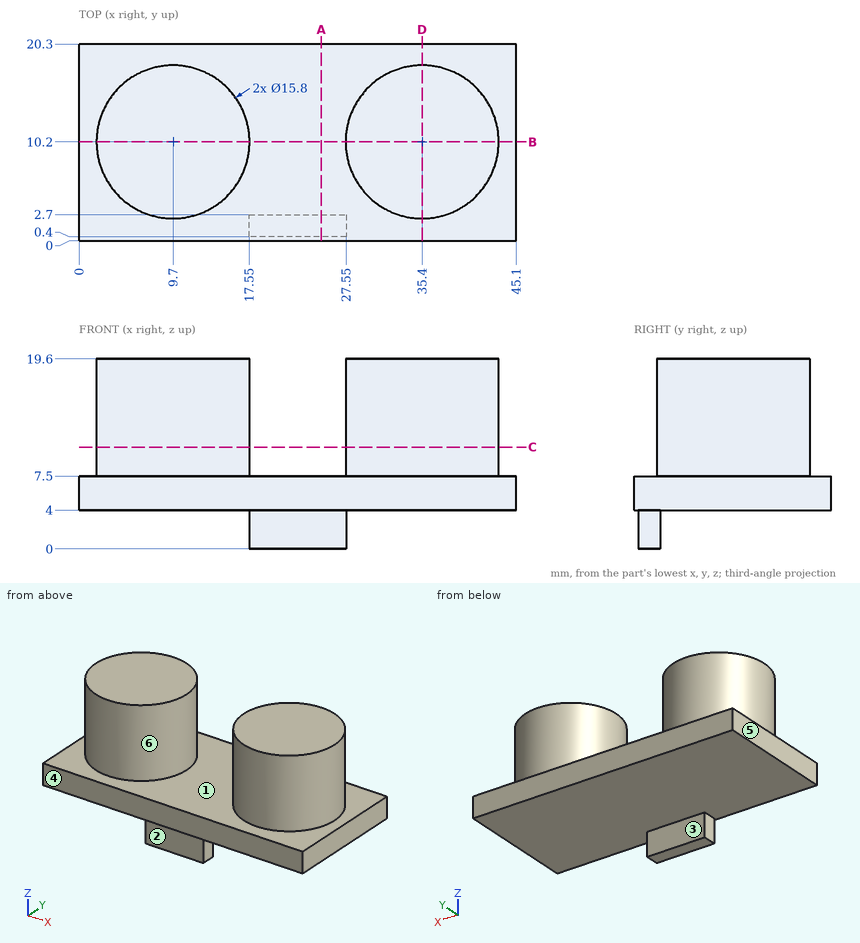
Geometry: see drawing. Coordinates: mm, zero at the bounding-box minimum. A direction names the side the tool comes from. Give positions to 0.01 mm unless a question says otherwise; leave off trailing zeros. Write each loop counter-clockwise with the first axis right and the second up, starting at its lowest first coordinate (ties: lowest second). Pieces come first, ordered by that corner, then holes. Notation, with made-up numbers: (0, 73.25) - (40, 73.25) arc R12 ccw to (40, 89.25) - close; hole circle Ø4 at (38, 16). An arc over 180 degrees is marked (long way). Return JSON: item names as keys, results as strings. Group by question number.
1) First-contact query: P1, Ø3, axis at y = 14, z = 15.5, coming from the -X side; P2, Ø6, axis at x = 8.5, z = 9, coming from the -Y side; P3, Ø2, axis at x = 20.5, z = 1.5, coming from the +Y side; P4, Ø4.5, axis at x = 20.5, z = 1.5, coming from the -Y side. Flat tips, straight axial feed; report the tip coordinate or a pass-through.
2) Section C-C on z = 10.5. Return the cut outline in (x, y), plus the area to 3 significant figures.
3) Section A-A on x = 25. Return the cut outline in (y, z).
4) Section B-B on y = 10.2. Return the cut outline in (x, z), plus the area to 3 significant figures.
5) Line query: line 1 (Z direction, x = 13, y = 14.75); line 2 (Z direction, x = 25.5, y = 10.5); line 3 (X direction, y = 3.25, z = 16.5). Output: solid intervals per line, ascending.
6) Set-up query: the marked faces 1, 2 and 3. Return all of +Z, -Z, +X, -X, +Y, -Y with unobstructed straight access to the full face (end or side cutting, diameter ignored); none if empty.
7) Mould query, pull axis X, two halves, no side actions, for the marked faces 4, 5 and 6. Classes: released by +X, released by -X, zero draft, split by the parting line, or undercut.
8) Section D-D on x = 35.4. Return the cut outline in (y, z), plus the area to 3 significant figures.
Filled in:
{
 "1": {"P1": "stops at x = 2.14", "P2": "stops at y = 0", "P3": "stops at y = 2.7", "P4": "stops at y = 0.4"},
 "2": {"outline": "circle Ø15.8 at (9.7, 10.2); circle Ø15.8 at (35.4, 10.2)", "area": "392 mm^2"},
 "3": {"outline": "(0, 4) - (0.4, 4) - (0.4, 0) - (2.7, 0) - (2.7, 4) - (20.3, 4) - (20.3, 7.5) - (0, 7.5) - close"},
 "4": {"outline": "(0, 4) - (45.1, 4) - (45.1, 7.5) - (43.3, 7.5) - (43.3, 19.6) - (27.5, 19.6) - (27.5, 7.5) - (17.6, 7.5) - (17.6, 19.6) - (1.8, 19.6) - (1.8, 7.5) - (0, 7.5) - close", "area": "540 mm^2"},
 "5": {"line 1": "z = 4 to 19.6", "line 2": "z = 4 to 7.5", "line 3": "x = 5.94 to 13.46, 31.64 to 39.16"},
 "6": {"face 1": "+Z", "face 2": "-Z, +X, -X, -Y", "face 3": "-Z, +X, -X, +Y"},
 "7": {"face 4": "zero draft", "face 5": "released by -X", "face 6": "undercut"},
 "8": {"outline": "(0, 4) - (20.3, 4) - (20.3, 7.5) - (18.1, 7.5) - (18.1, 19.6) - (2.3, 19.6) - (2.3, 7.5) - (0, 7.5) - close", "area": "262 mm^2"}
}
